Work out the finished part from the listing and answer in its coordinate system (mm). A direction names the side the tool comes from. Give positions to 0.01 mm unless a question says otherwise; leave off trailing zeros. Write each loop counter-clockwise with the first axis right and the second up, starting at its lowest first coordinate (ties: lowest second). Pieces come first, ordered by that corner, then holes. Notation, with made-up numbers: (65, -38) -> (114, -38) arc R33 cw to (114, -6) -> close; hole circle Ø9 at (48.5, 54). An arc over 180 degrees is marked (long way). Write item = value, one per line. Start each with the question number.
from build123d import *

# Parameters (mm, degrees)
SKIZZE1_R                       = 11.75
AUFSATZ_LINEAR_AUSTRAGEN1_DEPTH = 10
SKIZZE2_R                       = 13
SKIZZE2_R_2                     = 11.75
AUFSATZ_LINEAR_AUSTRAGEN2_DEPTH = 5


with BuildPart() as part:
    # Skizze1 → Aufsatz-Linear austragen1 (new body)
    with BuildSketch(Plane(origin=(0, 0, 0), x_dir=(1, 0, 0), z_dir=(0, 1, 0))):
        Polygon((15.588457268, 0), (7.794228634, 13.5), (-7.794228634, 13.5), (-15.588457268, 0), (-7.794228634, -13.5), (7.794228634, -13.5), align=None)
        with Locations(Location((0, 0, 0), (0, 0, 270))):
            Circle(SKIZZE1_R, mode=Mode.SUBTRACT)
    extrude(amount=AUFSATZ_LINEAR_AUSTRAGEN1_DEPTH)

    # Skizze2 → Aufsatz-Linear austragen2 (add)
    with BuildSketch(Plane(origin=(0, 10, 0), x_dir=(1, 0, 0), z_dir=(0, 1, 0))):
        with Locations(Location((0, 0, 0), (0, 0, 270))):
            Circle(SKIZZE2_R)
        with Locations(Location((0, 0, 0), (0, 0, 270))):
            Circle(SKIZZE2_R_2, mode=Mode.SUBTRACT)
    extrude(amount=AUFSATZ_LINEAR_AUSTRAGEN2_DEPTH)

    # Skizze3 → Rotation1 (revolve)
    with BuildSketch(Plane.XY, mode=Mode.PRIVATE) as rotation1_sk:
        with BuildLine():
            Line((-13, 15), (-11.75, 15))
            ThreePointArc((-11.75, 15), (-10.798097039, 17.298097039), (-8.5, 18.25))
            Line((-8.5, 18.25), (-7.25, 18.25))
            Line((-7.25, 18.25), (-7.25, 19.5))
            Line((-7.25, 19.5), (-8.5, 19.5))
            ThreePointArc((-8.5, 19.5), (-11.681980515, 18.181980515), (-13, 15))
        make_face()
    revolve(rotation1_sk.sketch.rotate(Axis((0, 0, 0), (0, 1, 0)), 270), axis=Axis((0, 0, 0), (0, 1, 0)))


solid = part.part
(1) Each of these flat-tipped pins is pushed along its axis until it touches: pin 1 (2 mm diameter, centred on x = 7.5, y = 12.5, fed in from +Z); pin 2 (5 mm diameter, centred on x = -3, y = 14, fed in from -Z); pin 3 (1 mm diameter, centred on y = 8.5, z = 3, fed in from +X); pin 4 (8 mm diameter, centred on x = -3.5, z = -5.5, fed in from +Y). Where does it stop, or does it pass through?
(2) For faces 5 (the cylindrical face through (2.777, 18.884, -6.697)), 6 (the flat face through (13, 10, -4)), determine the directions among +Z, -Z, +X, -X, +Y, -Y from which every point of the face is accessible in a straight line to the end or side of a thin tool.
(3) A cutting plane is placed at B-B, the plane y = 5.25. Write down the section's boundary in (x, z).
(4) A cutting plane is placed at C-C, the plane y = 12. Write down the section's boundary in (x, z).
(5) Determine the mould class of faces 1 (the cylindrical face through (-7.91, 12.465, -10.316)), 2 (the flat face through (-3, 18.25, -7)), 3 (the cylindrical face through (7.9, 7.4, -8.7)), 4 (the flat face through (0, 5, -13.5)) for opening direction Z: pulls with the +Z half, pulls with the -Z half, needs draft (parallel to the pull), parting line crosses it, or undercut.
(6) Find the intervals of material crossed by line 1 along X through (y, z) = (10.5, 0); line 2 along X through (y, z) = (8.5, 0); line 3 along Z through (x, y) = (5, 2), in increasing order.
(7) A cutting plane is placed at A-A, the plane x = 0. Write down the section's boundary in (y, z).
Results list:
q1.pin_1 = 11.26
q1.pin_2 = -12.99
q1.pin_3 = 14.15
q1.pin_4 = 19.5
q2.face_5 = +Y, -Y
q2.face_6 = +Y
q3.outline = (-15.59, 0) -> (-7.79, -13.5) -> (7.79, -13.5) -> (15.59, 0) -> (7.79, 13.5) -> (-7.79, 13.5) -> close; hole circle Ø23.5 at (0, 0)
q4.outline = circle Ø26 at (0, 0); hole circle Ø23.5 at (0, 0)
q5.face_1 = parting line crosses it
q5.face_2 = undercut
q5.face_3 = undercut
q5.face_4 = pulls with the -Z half
q6.line_1 = -13 to -11.75, 11.75 to 13
q6.line_2 = -15.59 to -11.75, 11.75 to 15.59
q6.line_3 = -13.5 to -10.63, 10.63 to 13.5
q7.outline = (0, -13.5) -> (10, -13.5) -> (10, -13) -> (15, -13) arc R4.5 ccw to (19.5, -8.5) -> (19.5, -7.25) -> (18.25, -7.25) -> (18.25, -8.5) arc R3.25 cw to (15, -11.75) -> (0, -11.75) -> close; (0, 11.75) -> (15, 11.75) arc R3.25 cw to (18.25, 8.5) -> (18.25, 7.25) -> (19.5, 7.25) -> (19.5, 8.5) arc R4.5 ccw to (15, 13) -> (10, 13) -> (10, 13.5) -> (0, 13.5) -> close
